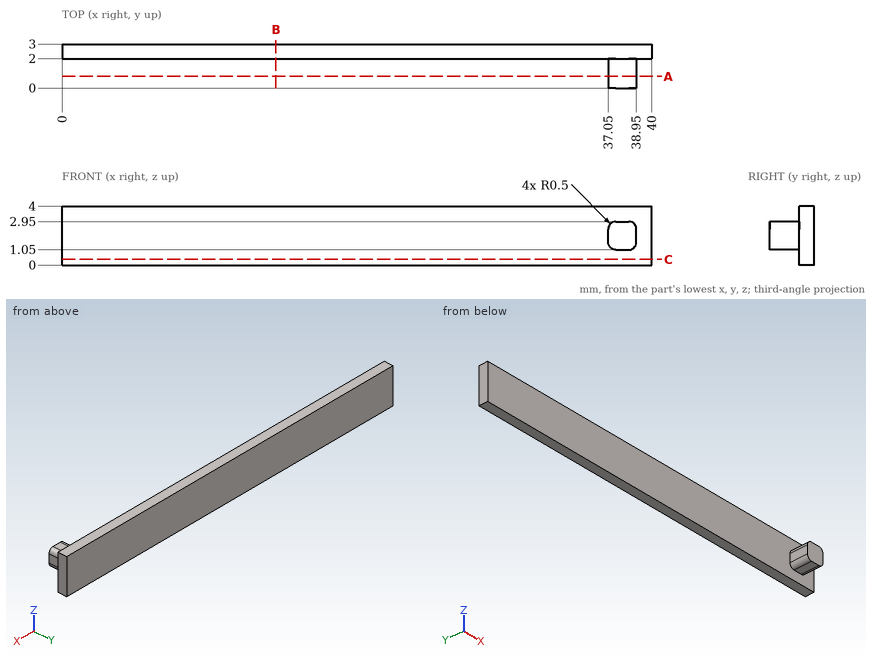
Design review of the part shown in the three views and the two pictorial views. Dimensions are in mm from the part's minimum x, y and z. Coordinates: 2 decimals unless noted, no trailing zeros. Write each loop counter-clockwise with the first axis right and the second up, starting at its lowest first coordinate (ties: lowest second). Pieces come first, ordered by that corner, then holes. Notation, with made-up numbers: (-37, -12.5) -> (17, -12.5) arc R18 cw to (17, 12.5) -> close; hole circle Ø9 at (12, -18.75). An arc over 180 degrees is marked (long way). Answer in a Markdown table with one row per item.
1. We need section A-A, the plane y = 0.8. State the section outline as (x, z) points.
Answers below:
| item | result |
|---|---|
| outline | (37.05, 1.55) arc R0.5 ccw to (37.55, 1.05) -> (38.45, 1.05) arc R0.5 ccw to (38.95, 1.55) -> (38.95, 2.45) arc R0.5 ccw to (38.45, 2.95) -> (37.55, 2.95) arc R0.5 ccw to (37.05, 2.45) -> close |
2. Wall thickness on probe 1 along Y at (x, z) = (20.5, 2.35); probe 2 along X at (y, z) = (0.2, 2.25); probe 3 along Z at (x, y) = (38, 1): over which ranges is each line inside the solid? List them lowest first. Write a range as [from, to].
Answers below:
| item | result |
|---|---|
| probe 1 | y = [2, 3] |
| probe 2 | x = [37.05, 38.95] |
| probe 3 | z = [1.05, 2.95] |
3. We need section C-C, the plane z = 0.4. State the section outline as (x, y) points, and give its area (3 significant figures).
Answers below:
| item | result |
|---|---|
| outline | (0, 2) -> (40, 2) -> (40, 3) -> (0, 3) -> close |
| area | 40.0 mm^2 |
4. Clearance check with flat-ended pins moving along their axes: pin 1 Ø1 at (x, y) = (38, 1) entering from -Z; pin 2 Ø1 at (y, z) = (0.5, 2) entering from +X; pin 3 Ø0.7 at (x, y) = (38, 1.5) entering from +Z. State where each tip first meets the part, or that it passes through.
Answers below:
| item | result |
|---|---|
| pin 1 | stops at z = 1.05 |
| pin 2 | stops at x = 38.95 |
| pin 3 | stops at z = 2.95 |
5. We need section B-B, the plane x = 14.5. State the section outline as (y, z) points.
Answers below:
| item | result |
|---|---|
| outline | (2, 0) -> (3, 0) -> (3, 4) -> (2, 4) -> close |
